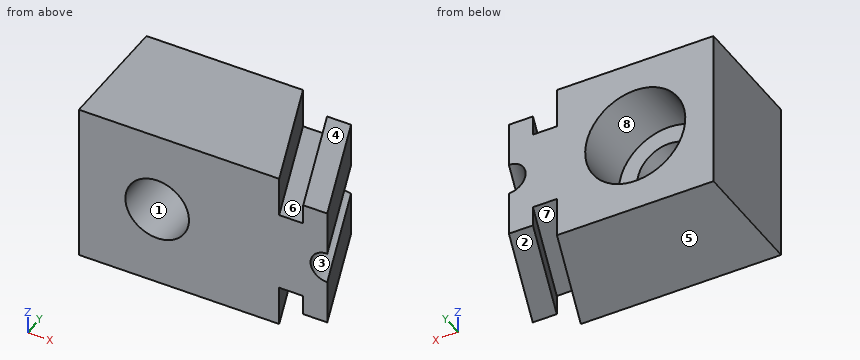
Autodesk Inventor part; units mm, degrees
ref_plane "Work Plane3" through (39.37, 0, 0) normal (-0.342, 0.9397, 0) x (0, 0, -1)
ref_plane "YZ Plane" through (0, 0, 0) normal (1, 0, 0) x (0, 1, 0)
ref_plane "XZ Plane" through (0, 0, 0) normal (0, 1, 0) x (-1, 0, 0)
sketch "Sketch1" plane through (0, 0, 0) normal (0, 1, 0) x (-1, 0, 0)
  line L0 (0, 0) -> (-39.37, 0)
  line L1 (-39.37, 0) -> (-39.37, -25.4)
  line L2 (-39.37, -25.4) -> (0, -25.4)
  line L3 (0, -25.4) -> (0, 0)
  line L4 (-35.56, -25.4) -> (-35.56, 0)
  line L5 (0, -12.7) -> (-39.37, -12.7) construction
  line L6 (-31.75, -25.4) -> (-31.75, 0)
  line L7 (-31.75, -19.05) -> (-35.56, -19.05)
  line L8 (-31.75, -6.35) -> (-35.56, -6.35)
  line L9 (-35.56, -22.225) -> (-39.37, -22.225)
  line L10 (-35.56, -3.175) -> (-39.37, -3.175)
  point P0 (-35.56, -6.35)
  point P1 (-39.37, -3.175)
  dimension "d7" = 25.4
  dimension "d10" = 3.81
  dimension "d34" = 3.81
  dimension "d35" = 12.7
  dimension "d36" = 19.05
  dimension "d37" = 31.75
extrude "Extrusion1" add sketch "Sketch1" along normal blind 19.05
sketch "Sketch3" plane through (0, 0, 0) normal (0, 0, 1) x (1, 0, 0)
  line L0 (0, 0) -> (39.37, 0)
  line L1 (39.37, 0) -> (39.37, 19.05)
  line L2 (0, 19.05) -> (39.37, 19.05)
  line L3 (0, 0) -> (0, 19.05)
  line L4 (24.8164, 19.05) -> (31.75, 0)
  dimension "d14" = 70
  dimension "d15" = 31.75
sweep "Sweep1" cut profiles "Sketch1" path "Sketch3" path curves L4 contours L6 L8 L4 L0 | L4 L10 L1 L0 | L2 L4 L7 L6 | L2 L1 L9 L4
ref_plane "Work Plane3" through (39.37, 0, 0) normal (-0.342, 0.9397, 0) x (0, 0, -1)
ref_plane "Work Plane2" through (39.37, 0, 0) normal (-0.9397, -0.342, 0) x (0, 0, -1)
sketch "Sketch5" plane through (39.37, 0, 0) normal (-0.342, 0.9397, 0) x (0, 0, -1)
  point P0 (12.7, 0)
hole "Hole2" at (39.37, 0, -12.7) direction (-0.342, 0.9397, 0) diameter 4.9784 end through all
split "Split1" plane through (39.37, 0, 0) removes the side toward (0.9397, 0.342, 0)
sketch "Sketch4" plane through (0, 19.05, 0) normal (0, 1, 0) x (1, 0, 0)
  line L0 (32.4364, 15.1892) -> (32.4364, 22.225)
  line L1 (32.4364, 22.225) -> (28.6264, 22.225)
  line L2 (28.6264, 22.225) -> (28.6264, 19.05)
  line L3 (28.6264, 19.05) -> (24.8164, 19.05)
  line L4 (24.8164, 19.05) -> (24.8164, 25.4)
  line L5 (24.8164, 25.4) -> (0, 25.4)
  line L6 (0, 25.4) -> (0, 0)
  line L7 (0, 0) -> (24.8164, 0)
  line L8 (24.8164, 0) -> (24.8164, 6.35)
  line L9 (24.8164, 6.35) -> (28.6264, 6.35)
  line L10 (28.6264, 6.35) -> (28.6264, 3.175)
  line L11 (28.6264, 3.175) -> (32.4364, 3.175)
  line L12 (32.4364, 3.175) -> (32.4364, 10.2108)
  ellipse E0 centre (32.4364, 12.7) end of major axis (29.7874, 12.7) minor radius 2.4892 (32.4364, 15.1892) -> (32.4364, 10.2108) ccw
  point P0 (12.4082, 12.7)
  point P1 (0, 12.7)
  point P2 (12.4082, 25.4)
hole "Hole1" at (12.4082, 19.05, -12.7) direction (0, -1, 0) diameter 10.0838 end through all counterbore diameter 15.875 counterbore depth 9.525
equation "\"d10\" = d34"
equation "\"d34\" = slotWidth"
equation "\"d14\" = slopeAngle"
equation "\"d18\" = slopeAngle"
equation "\"slopeAngle\" = 70deg"
equation "\"slotWidth\" = 3.81"
properties material "Steel, Alloy"
Geometry check sheet. Reference: the model listing, model coordinates, mm. Face numbers are marked on the shaded views. A direction names the side the tool comes from. Give positions to 0.01 mm unless a question says otherwise; leave off trailing zeros. Order: outer loops, then holes, each group sorted by start corner. A loop starts at its lowest first (then second) coordinate and runs counter-clockwise, first axis right, second up.
1. Access from +Z, -Z, +X, -X, +Y, -Y to the whole of each face (thin tool, end or side, straight path). Record for the marked faces 4, 5, 6, 7 and 8.
2. Section check D-D, the plane z = -23. Enter the section's corners in (x, y).
3. Thickness scan on L1, parallel to Y at x = 20, z = -11.25 (3 decimals); L2, parallel to X at y = 4.75, z = -21; L3, parallel to X at y = 7, z = -6. Record the ranges inside material, lowest first.
4. Gauge pin test, flat ends, axial feed: pin 1 Ø5 at (x, z) = (15, -15.5) entering from +Y (3 decimals); pin 2 Ø5 at (y, z) = (11.5, -18.5) entering from +X; pin 3 Ø8 at (y, z) = (5.5, -14.5) entering from +X. Record the tip position at first contact, or that the pin passes through.
5. Section check A-A, the plane z = -4.25. Enter the section's corners in (x, y).
6. Section check C-C, the plane z = -12.7. Enter the section's corners in (x, y) (3 decimals).
7. Section check B-B, the plane x = 13. Enter the section's corners in (y, z) (3 decimals).
8. Release check for a two-part mould opening along X. For the marked faces 1, 2 and 3 record: pulls with the +X half, pulls with the -X half, needs draft (parallel to the pull), parting line crosses it, or undercut.
Values follow:
1. face 4: +Z, +X, +Y
1. face 5: -Z, +X, -X, +Y, -Y
1. face 6: +Z
1. face 7: -Z
1. face 8: +Y
2. outline: (0, 0) - (31.75, 0) - (24.82, 19.05) - (0, 19.05) - close
3. L1: y = 0 to 9.525
3. L2: x = 0 to 30.02, 33.83 to 37.64
3. L3: x = 0 to 29.2, 33.01 to 36.82
4. pin 1: stops at y = 9.525
4. pin 2: stops at x = 36.09
4. pin 3: stops at x = 38.8
5. outline: (0, 0) - (31.75, 0) - (24.82, 19.05) - (0, 19.05) - close; (28.63, 19.05) - (35.56, 0) - (39.37, 0) - (32.44, 19.05) - close
6. outline: (0, 0) - (7.366, 0) - (7.366, 9.525) - (4.471, 9.525) - (4.471, 19.05) - (0, 19.05) - close; (17.45, 0) - (36.721, 0) - (29.787, 19.05) - (20.346, 19.05) - (20.346, 9.525) - (17.45, 9.525) - close
7. outline: (0, -25.4) - (19.05, -25.4) - (19.05, -20.615) - (9.525, -20.615) - (9.525, -17.707) - (0, -17.707) - close; (0, -7.693) - (9.525, -7.693) - (9.525, -4.785) - (19.05, -4.785) - (19.05, 0) - (0, 0) - close
8. face 1: undercut
8. face 2: needs draft
8. face 3: pulls with the +X half
